Part model, mm, in its own coordinate system. A direction names the side the tool comes from. Round coordinates to 2 decimals unless told otherwise and drop trailing zeros. Write each loop counter-clockwise with the first axis right and the second up, starting at its lowest first coordinate (ties: lowest second). Pieces come first, ordered by that corner, then holes.
```python
from build123d import *

# Parameters (mm, degrees)
F0_W      = 200
F0_H      = 80
F1_DEPTH  = 10
F2_W      = 42
F2_H      = 21
F3_DEPTH  = 10.001
F4_W      = 71
F4_H      = 24.5
F5_DEPTH  = 10.001
F6_R      = 3.5
F7_DEPTH  = 10.001
F8_R      = 5
F11_W     = 70
F11_H     = 20
F11_H_2   = 40
F9_W      = 12.4
F9_H      = 11.4
F12_DEPTH = 10.001
F13_R     = 5


with BuildPart() as f1:
    # F0 (on Top) → F1 (new body)
    with BuildSketch(Plane.XY):
        Rectangle(F0_W, F0_H)
    extrude(amount=F1_DEPTH)

    # F2 (on face) → F3 (cut, through all)
    with BuildSketch(Plane.XY.offset(10)):
        with Locations((-55, 10)):
            Rectangle(F2_W, F2_H)
    extrude(amount=-F3_DEPTH, mode=Mode.SUBTRACT)

    # F4 (on face) → F5 (cut, through all)
    with BuildSketch(Plane.XY.offset(10)):
        with BuildLine():
            Line((-78.9, 12.85), (-78.9, 15.1))
            Line((-78.9, 15.1), (-76.65, 15.1))
            ThreePointArc((-76.65, 15.1), (-80.4909902577, 16.6909902577), (-78.9, 12.85))
        make_face()
        with BuildLine():
            Line((-76.65, 15.1), (-78.9, 15.1))
            Line((-78.9, 15.1), (-78.9, 12.85))
            ThreePointArc((-78.9, 12.85), (-77.3090097423, 13.5090097423), (-76.65, 15.1))
        make_face()
        with BuildLine():
            Line((-78.9, 4.9), (-78.9, 7.15))
            ThreePointArc((-78.9, 7.15), (-80.4909902577, 3.3090097423), (-76.65, 4.9))
            Line((-76.65, 4.9), (-78.9, 4.9))
        make_face()
        with BuildLine():
            ThreePointArc((-76.65, 4.9), (-77.3090097423, 6.4909902577), (-78.9, 7.15))
            Line((-78.9, 7.15), (-78.9, 4.9))
            Line((-78.9, 4.9), (-76.65, 4.9))
        make_face()
        with BuildLine():
            Line((-31.1, 15.1), (-33.35, 15.1))
            ThreePointArc((-33.35, 15.1), (-32.6909902577, 13.5090097423), (-31.1, 12.85))
            Line((-31.1, 12.85), (-31.1, 15.1))
        make_face()
        with BuildLine():
            ThreePointArc((-28.85, 15.1), (-31.1, 17.35), (-33.35, 15.1))
            Line((-33.35, 15.1), (-31.1, 15.1))
            Line((-31.1, 15.1), (-31.1, 12.85))
            ThreePointArc((-31.1, 12.85), (-29.5090097423, 13.5090097423), (-28.85, 15.1))
        make_face()
        with BuildLine():
            ThreePointArc((-31.1, 7.15), (-32.6909902577, 6.4909902577), (-33.35, 4.9))
            Line((-33.35, 4.9), (-31.1, 4.9))
            Line((-31.1, 4.9), (-31.1, 7.15))
        make_face()
        with BuildLine():
            Line((-31.1, 4.9), (-33.35, 4.9))
            ThreePointArc((-33.35, 4.9), (-31.1, 2.65), (-28.85, 4.9))
            ThreePointArc((-28.85, 4.9), (-29.5090097423, 6.4909902577), (-31.1, 7.15))
            Line((-31.1, 7.15), (-31.1, 4.9))
        make_face()
        with Locations((-54.5, -21.75)):
            Rectangle(F4_W, F4_H)
    extrude(amount=-F5_DEPTH, mode=Mode.SUBTRACT)

    # F6 (on face) → F7 (cut, through all)
    with BuildSketch(Plane.XY.offset(10)):
        with Locations((-88.3175069503, 30)):
            Circle(F6_R)
        with Locations((12.1812492609, 30)):
            Circle(F6_R)
    extrude(amount=-F7_DEPTH, mode=Mode.SUBTRACT)

    # F8
    f8_edges = [f1.edges().sort_by_distance(p)[0] for p in [
        (-100, 40, 5),
        (-100, -40, 5),
        (100, 40, 5),
        (100, -40, 5),
    ]]
    fillet(f8_edges, radius=F8_R)

    # F11 (on face) + F10 (on face) + F9 (on face) → F12 (cut, through all)
    with BuildSketch(Plane.XY.offset(10)):
        with Locations((65, 30)):
            Rectangle(F11_W, F11_H)
        with Locations((65, -20)):
            Rectangle(F11_W, F11_H_2)
    with BuildSketch(Plane.XY.offset(10)):
        with BuildLine():
            ThreePointArc((96.425, 10), (94, 12.425), (91.575, 10))
            Line((91.575, 10), (94, 10))
            Line((94, 10), (94, 7.575))
            ThreePointArc((94, 7.575), (95.7147339444, 8.2852660556), (96.425, 10))
        make_face()
        with BuildLine():
            Line((94, 10), (91.575, 10))
            ThreePointArc((91.575, 10), (92.2852660556, 8.2852660556), (94, 7.575))
            Line((94, 7.575), (94, 10))
        make_face()
    with BuildSketch(Plane.XY.offset(10)):
        with Locations((6.2, -25.7)):
            Rectangle(F9_W, F9_H)
    extrude(amount=-F12_DEPTH, mode=Mode.SUBTRACT)

    # F13
    f13_edges = [f1.edges().sort_by_distance(p)[0] for p in [
        (30, 40, 5),
        (30, 20, 5),
        (100, 20, 5),
        (30, -40, 5),
        (100, 0, 5),
        (30, 0, 5),
    ]]
    fillet(f13_edges, radius=F13_R)


solid = f1.part
```
Q1. Cut at D-D on z = 6.5. State how many separate pieces and enclosed holes the cut face has, plus the area to 3 significant figures.
Values follow:
separate pieces: 1
enclosed holes: 10
area: 8,860 mm2
Q2. Cut at B-B on y = -23.5. Write the cut outline in (x, z), plus the area to 3 significant figures.
Values follow:
outline: (-100, 0) - (-90, 0) - (-90, 10) - (-100, 10) - close; (-19, 0) - (0, 0) - (0, 10) - (-19, 10) - close; (12.4, 0) - (30, 0) - (30, 10) - (12.4, 10) - close
area: 466 mm2
Q3. Which spindle directions (+Z, -Z, +X, -X, +Y, -Y) get a long thin tool onto all of the face, cutting with end or side? Do faces 1 (the flat face through (65, 0, 5)), 2 (the flat face through (30, 30, 5)), 3 (the cylindrical face through (-99, -38, 5)), 4 (the flat face through (-19, -22, 5)). Say none if no direction does.
Values follow:
face 1: +Z, -Z, +X, -Y
face 2: +Z, -Z, +X, +Y
face 3: +Z, -Z, -X, -Y
face 4: +Z, -Z
Q4. Cut at A-A on y = 30. Write the cut outline in (x, z), plus the area to 3 significant figures.
Values follow:
outline: (-100, 0) - (-91.82, 0) - (-91.82, 10) - (-100, 10) - close; (-84.82, 0) - (8.68, 0) - (8.68, 10) - (-84.82, 10) - close; (15.68, 0) - (30, 0) - (30, 10) - (15.68, 10) - close
area: 1,160 mm2
Q5. Wall check: L1, parallel to Y at x = -68.5, z = 6; L2, parallel to X at y = -24, z = 8.5; L3, parallel to X at y = 4.9, z = 2.5. Give the ranges that are in metal, low to high.
Values follow:
L1: y = -40 to -34, -9.5 to -0.5, 20.5 to 40
L2: x = -100 to -90, -19 to 0, 12.4 to 30
L3: x = -100 to -81.15, -76.65 to -76, -34 to -33.35, -28.85 to 100
Q6. Cut at C-C on x = 82. Write the cut outline in (y, z).
Values follow:
outline: (0, 0) - (20, 0) - (20, 10) - (0, 10) - close
Q7. Mould opens along X. For faces 5 (the cylindrical face through (29, -38, 5)), 6 (the flat face through (12.4, -26, 5)), 7 (the cylindrical face through (-99, 38, 5)) say: +X half, -X half, draft (parallel to the pull), parting line (faces both ways), or undercut.
Values follow:
face 5: +X half
face 6: undercut
face 7: -X half
Q8. Drop flat-ended pins along their axis: pin 1 (3 mm diameter, centred on y = -23, z = 4, fed in from +X); pin 2 (5 mm diameter, centred on x = 70.5, z = 5.5, fed in from -Y); pin 3 (1.5 mm diameter, centred on x = 19.5, y = 19, fed in from -Z); pin 4 (1.5 mm diameter, centred on x = 43.5, z = 4, fed in from +Y). Give the stop position or say it passes through.
Values follow:
pin 1: stops at x = 30
pin 2: stops at y = 0
pin 3: stops at z = 0
pin 4: stops at y = 20
